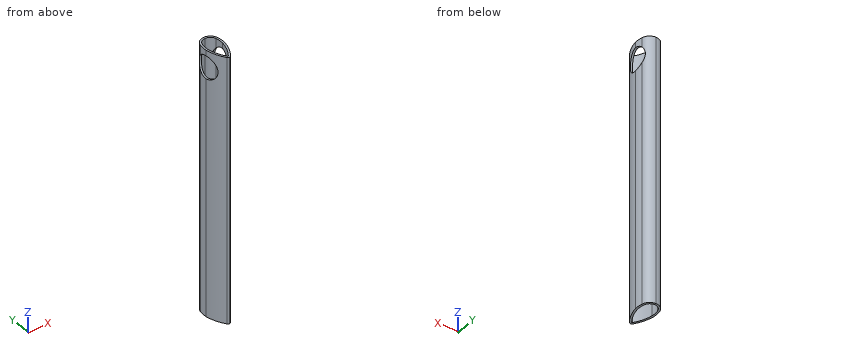
from build123d import *

# Parameters (mm, degrees)
F1_DEPTH = 50
F2_R     = 15.0073664172
F3_DEPTH = 25
F4_DEPTH = 300


# Not quite as in the source:
# - ends of sketch curves that miss each other by under 0.0002 mm in the source are joined


with BuildPart() as f1:
    # F0 (on Top) → F1 (new body)
    with BuildSketch(Plane.XY):
        with BuildLine():
            ThreePointArc((11.5946267397, 13.5320293348), (7.4846115717, 20.3323038327), (0, 22.9999896369))
            ThreePointArc((0, 22.9999896369), (-7.4846118013, 20.3323037509), (-11.5946270955, 13.5320290443))
            ThreePointArc((-11.5946270955, 13.5320290443), (-12.4147063987, 7.922168163), (-12.3388696742, 2.2531896672))
            ThreePointArc((-12.3388696742, 2.2531896672), (-8.8719983331, -10.2277960598), (-2.5843411657, -21.5529706895))
            ThreePointArc((-2.5843411657, -21.5529706895), (-1.4841666884, -22.619355112), (7e-08, -22.9998983316))
            ThreePointArc((7e-08, -22.9998983316), (1.4841670374, -22.6193504592), (2.5843454149, -21.5529672416))
            ThreePointArc((2.5843454149, -21.5529672416), (8.872000694, -10.2277939953), (12.3388707315, 2.2531898872))
            ThreePointArc((12.3388707315, 2.2531898872), (12.4147117976, 7.9221688824), (11.5946267397, 13.5320293348))
        make_face()
        with BuildLine():
            ThreePointArc((0, 20.5299898954), (5.9328912698, 18.410508519), (9.1798866708, 13.011580756))
            ThreePointArc((9.1798866708, 13.011580756), (9.9466025789, 7.8114966866), (9.8862458377, 2.5555396209))
            ThreePointArc((9.8862458377, 2.5555396209), (6.5447373666, -9.3927265107), (0.4963170659, -20.2252402669))
            ThreePointArc((0.4963170659, -20.2252402669), (0.2950851675, -20.4538524641), (4.0013e-05, -20.529391662))
            ThreePointArc((4.0013e-05, -20.529391662), (-0.2950640986, -20.4538699373), (-0.4963311707, -20.2252183832))
            ThreePointArc((-0.4963311707, -20.2252183832), (-6.5447290925, -9.3927429052), (-9.8862348466, 2.5554779538))
            ThreePointArc((-9.8862348466, 2.5554779538), (-9.9466064803, 7.8113582927), (-9.1799291893, 13.0113706774))
            ThreePointArc((-9.1799291893, 13.0113706774), (-5.9329742724, 18.4104406446), (0, 20.5299898954))
        make_face(mode=Mode.SUBTRACT)
    extrude(amount=F1_DEPTH)

    # F2 (on Right) → F3 (cut, symmetric)
    with BuildSketch(Plane.YZ):
        with Locations((2.2132990416, 27.6111345738)):
            Circle(F2_R)
    extrude(amount=F3_DEPTH, both=True, mode=Mode.SUBTRACT)

    # F4 (add): a face of the model
    f4_faces = [f1.faces().sort_by_distance(p)[0] for p in [
        (7.153517518, 19.9268403702, 0),
    ]]
    extrude(f4_faces, amount=F4_DEPTH)


solid = f1.part
The model under review builds one solid part; all positions refer to its coordinate system, in mm. Give positions to 0.01 mm unless a question says otherwise; leave off trailing zeros. Loops run counter-clockwise (first coordinate to the right, second up) from the corner with the lowest first, then second, coordinate; pieces in that order, holes last. Notation, with made-up numbers: (19, 17.25) -> (44, 17.25) arc R9 cw to (44, 32.25) -> close; hole circle Ø7 at (37, 61.25). An arc over 180 degrees is marked (long way). Answer as a JSON object with one key per item and string values. Group by question number.
Q1. Insertion check: pin 1 (2 mm diameter, centred on y = -14.5, z = 13, fed in from -X) (3 decimals); pin 2 (5 mm diameter, centred on y = -17, z = -213.5, fed in from +X); pin 3 (10 mm diameter, centred on x = 6, z = -260.5, fed in from +Y). Each pin has a flat end and moves straight along its axis. Give the tip position at first contact, or say it passes through.
Q2. Take a section at C-C (y = 6). Write out the cut boundary in (x, z), plus the area to 3 significant figures.
Q3. Take a section at A-A (y = -8). Write out the cut boundary in (x, z).
Q4. Take a section at B-B (z = -217). Write out the cut boundary in (x, y).
Q5. Wall thickness on line 1 along X through (y, z) = (7, -2); line 2 along Z through (x, y) = (10.75, 4); line 3 along X through (y, z) = (-9, -209): over which ranges is each line inside the solid? List them lowest first.
Answer below:
{
 "1": {"pin 1": "stops at x = -7.405", "pin 2": "stops at x = 6.9", "pin 3": "stops at y = 22.96"},
 "2": {"outline": "(-12.49, -300) -> (-10.02, -300) -> (-10.02, 13.09) -> (-12.49, 13.09) -> close; (-12.49, 42.13) -> (-10.02, 42.13) -> (-10.02, 50) -> (-12.49, 50) -> close; (10.02, -300) -> (12.49, -300) -> (12.49, 13.09) -> (10.02, 13.09) -> close; (10.02, 42.13) -> (12.49, 42.13) -> (12.49, 50) -> (10.02, 50) -> close", "area": "1,590 mm2"},
 "3": {"outline": "(-9.73, -300) -> (-7.1, -300) -> (-7.1, 16.62) -> (-9.73, 16.62) -> close; (-9.73, 38.61) -> (-7.1, 38.61) -> (-7.1, 50) -> (-9.73, 50) -> close; (7.1, -300) -> (9.73, -300) -> (9.73, 16.62) -> (7.1, 16.62) -> close; (7.1, 38.61) -> (9.73, 38.61) -> (9.73, 50) -> (7.1, 50) -> close"},
 "4": {"outline": "(-12.34, 2.25) arc R55.04 ccw to (-2.58, -21.55) arc R2.99 ccw to (0, -23) arc R2.99 ccw to (2.58, -21.55) arc R55.04 ccw to (12.34, 2.25) arc R35.8 ccw to (11.59, 13.53) arc R11.83 ccw to (-11.59, 13.53) arc R35.8 ccw to start; hole (-9.89, 2.56) arc R52.57 ccw to (-0.5, -20.23) arc R0.52 ccw to (0, -20.53) arc R0.52 ccw to (0.5, -20.23) arc R52.57 ccw to (9.89, 2.56) arc R33.33 ccw to (9.18, 13.01) arc R9.36 ccw to (-9.18, 13.01) arc R33.33 ccw to start"},
 "5": {"line 1": "x = -12.46 to -9.99, 9.99 to 12.46", "line 2": "z = -300 to 12.71, 42.51 to 50", "line 3": "x = -9.36 to -6.7, 6.7 to 9.36"}
}
